The model under review builds one solid part; all positions refer to its coordinate system, in mm. Face numbers are marked on the shaded views. A direction names the side the tool comes from. Coordinates: 2 decimals unless noted, no trailing zeros. Write each loop counter-clockwise with the first axis right and the second up, starting at its lowest first coordinate (ties: lowest second). Pieces come first, ordered by that corner, then holes.
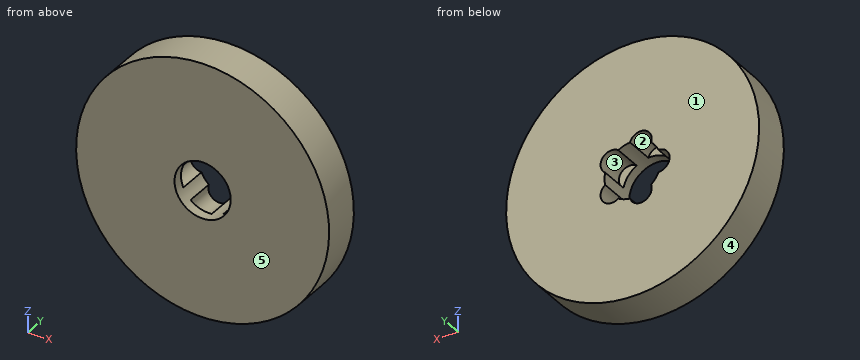
```python
from build123d import *

# Parameters (mm, degrees)
SKETCH1_R           = 22.5
BOSS_EXTRUDE1_DEPTH = 7
SKETCH2_R           = 5
CUT_EXTRUDE1_DEPTH  = 33.580669115
SKETCH3_R           = 1.981426301
CUT_EXTRUDE2_DEPTH  = 5.165946
CIRPATTERN1_START   = 1.834054269
CIRPATTERN1_DEPTH   = 5.165945731


# Read off the part's stored shape, not the designer's step: CirPattern1
with BuildPart() as part:
    # Sketch1 → Boss-Extrude1 (new body)
    with BuildSketch(Plane(origin=(0, 0, 0), x_dir=(1, 0, 0), z_dir=(0, 1, 0))):
        with Locations(Location((0, 0, 0), (0, 0, 270))):
            Circle(SKETCH1_R)
    extrude(amount=BOSS_EXTRUDE1_DEPTH)

    # Sketch2 → Cut-Extrude1 (cut, through all)
    with BuildSketch(Plane(origin=(0, 0, 0), x_dir=(1, 0, 0), z_dir=(0, 1, 0))):
        with Locations(Location((0, 0, 0), (0, 0, 270))):
            Circle(SKETCH2_R)
    extrude(amount=CUT_EXTRUDE1_DEPTH, mode=Mode.SUBTRACT)

    # Sketch3 → Cut-Extrude2 (cut)
    with BuildSketch(Plane(origin=(0, 7, 0), x_dir=(1, 0, 0), z_dir=(0, 1, 0))):
        with Locations((-4.596235577, 0)):
            Circle(SKETCH3_R)
    extrude(amount=-CUT_EXTRUDE2_DEPTH, mode=Mode.SUBTRACT)

    # CirPattern1 outline → CirPattern1 (cut)
    with BuildSketch(Plane(origin=(0, 0, 0), x_dir=(1, 0, 0), z_dir=(0, 1, 0)).offset(CIRPATTERN1_START)):
        with BuildLine():
            ThreePointArc((0.465854922, -4.978250616), (-1.545084972, -4.755282581), (-3.303026843, -3.753666697))
            ThreePointArc((-3.303026843, -3.753666697), (-2.032609304, -6.255728191), (0.465854922, -4.978250616))
        make_face()
        with BuildLine():
            ThreePointArc((0.465854922, 4.978250616), (-2.032609304, 6.255728191), (-3.303026843, 3.753666697))
            ThreePointArc((-3.303026843, 3.753666697), (-1.545084972, 4.755282581), (0.465854922, 4.978250616))
        make_face()
        with BuildLine():
            ThreePointArc((4.878554776, -1.095309683), (4.045084972, -2.938926261), (2.549257745, -4.301312003))
            ThreePointArc((2.549257745, -4.301312003), (5.321440243, -3.866252647), (4.878554776, -1.095309683))
        make_face()
        with BuildLine():
            ThreePointArc((4.878554776, 1.095309683), (5.321440243, 3.866252647), (2.549257745, 4.301312003))
            ThreePointArc((2.549257745, 4.301312003), (4.045084972, 2.938926261), (4.878554776, 1.095309683))
        make_face()
    extrude(amount=CIRPATTERN1_DEPTH, mode=Mode.SUBTRACT)


solid = part.part
```
Item 1: Mouldability with a two-part tool opening along X and no side actions: class the marked faces 3, 4 and 5 as pulls with the +X half, pulls with the -X half, needs draft (parallel to the pull), parting line crosses it, or undercut.
Solved:
face 3: undercut
face 4: parting line crosses it
face 5: needs draft
Item 2: Take a section at B-B, the plane y = 1. Write out the cut boundary in (x, z).
Solved:
outline: circle Ø45 at (0, 0); hole circle Ø10 at (0, 0)
Item 3: Take a section at D-D, the plane y = 5.75. Write out the cut boundary in (x, z).
Solved:
outline: circle Ø45 at (0, 0); hole (-4.59, -1.98) arc R5 ccw to (-3.3, -3.75) arc R1.98 ccw (long way) to (0.47, -4.98) arc R5 ccw to (2.55, -4.3) arc R1.98 ccw (long way) to (4.88, -1.1) arc R5 ccw to (4.88, 1.1) arc R1.98 ccw (long way) to (2.55, 4.3) arc R5 ccw to (0.47, 4.98) arc R1.98 ccw (long way) to (-3.3, 3.75) arc R5 ccw to (-4.59, 1.98) arc R1.98 ccw (long way) to start
Item 4: For pin 1 (1.3 mm diameter, centred on x = -1.5, z = -4.5, fed in from +Y); pin 2 (3 mm diameter, centred on y = 2.5, z = 12, fed in from -X); pin 3 (4 mm diameter, centred on y = 3.5, z = -3, fed in from -X), all flat-tipped, find the tip position at first contact; note any pin that passes through.
Solved:
pin 1: stops at y = 1.83
pin 2: stops at x = -19.9
pin 3: stops at x = -22.48
Item 5: To check wall thickness, follow line 1 along X through (y, z) = (5.25, 0); line 2 along Z through (x, y) = (4, 1); line 3 along Z through (x, y) = (-2.5, 3.75). State the ranges of each line that lie inside material, in increasing order.
Solved:
line 1: x = -22.5 to -6.58, 5 to 22.5
line 2: z = -22.14 to -3, 3 to 22.14
line 3: z = -22.36 to -6.03, 6.03 to 22.36
Item 6: Machinability: for the marked faces 1 and 2, which of the approach directions +Z, -Z, +X, -X, +Y, -Y give a long, thin tool a straight path to every point of the face, cutting with its end or side? Answer none if there is none.
Solved:
face 1: +Z, -Z, +X, -X, +Y
face 2: +Y
Item 7: Take a section at C-C, the plane x = -2. Write out the cut boundary in (y, z), plus the area to 3 significant figures.
Solved:
outline: (0, -22.41) - (7, -22.41) - (7, -6.27) - (1.83, -6.27) - (1.83, -4.58) - (0, -4.58) - close; (0, 4.58) - (1.83, 4.58) - (1.83, 6.27) - (7, 6.27) - (7, 22.41) - (0, 22.41) - close
area: 232 mm2
Item 8: Take a section at A-A, the plane z = 0. Write out the cut boundary in (x, y), plus the area to 3 significant figures.
Solved:
outline: (-22.5, 0) - (-5, 0) - (-5, 1.83) - (-6.58, 1.83) - (-6.58, 7) - (-22.5, 7) - close; (5, 0) - (22.5, 0) - (22.5, 7) - (5, 7) - close
area: 237 mm2
